Read the model definition and answer for the solid it produces. Units are mm, in the model's axes. Face numbers are marked on the shaded views. A direction names the side the tool comes from. Round coordinates to 2 decimals unless told otherwise and drop trailing zeros. Write each loop counter-clockwise with the first axis right and the second up, starting at its lowest first coordinate (ties: lowest second). Pieces come first, ordered by that corner, then holes. Notation, with made-up numbers: (81.25, -21) -> (127.25, -21) arc R19 ccw to (127.25, 1) -> close; hole circle Ø5 at (-0.5, -4.75). An arc over 180 degrees is marked (long way). Return JSON: item names as keys, results as strings.
from build123d import *

# Parameters (mm, degrees)
SKETCH1_R           = 2.75
SKETCH1_W           = 25
SKETCH1_H           = 18
BOSS_EXTRUDE1_DEPTH = 3
CUT_EXTRUDE1_REACH  = 132.035
SKETCH3_R           = 2.75
SKETCH2_R           = 2.75
BOSS_EXTRUDE2_DEPTH = 6
FILLET1_R           = 3
BOSS_EXTRUDE5_DEPTH = 4.5
BOSS_EXTRUDE6_DEPTH = 4.5


with BuildPart() as part:
    # Sketch1 → Boss-Extrude1 (new body)
    with BuildSketch(Plane.XY):
        Polygon((7.071067812, 0), (42.928932188, 0), (50, 7.071067812), (50, 43.5), (45.5, 48), (45.5, 112.928932188), (38.428932188, 120), (11.571067812, 120), (4.5, 112.928932188), (4.5, 48), (0, 43.5), (0, 7.071067812), align=None)
        with Locations((7.1, 10)):
            Circle(SKETCH1_R, mode=Mode.SUBTRACT)
        with Locations(Location((42.9, 10, 0), (0, 0, 180))):
            Circle(SKETCH1_R, mode=Mode.SUBTRACT)
        with BuildLine():
            Line((19, 50.75), (19, 104))
            ThreePointArc((19, 104), (25, 110), (31, 104))
            Line((31, 104), (31, 50.75))
            ThreePointArc((31, 50.75), (25, 44.75), (19, 50.75))
        make_face(mode=Mode.SUBTRACT)
        with Locations((25, 17.5)):
            Rectangle(SKETCH1_W, SKETCH1_H, mode=Mode.SUBTRACT)
    extrude(amount=BOSS_EXTRUDE1_DEPTH)

    # Sketch3 → Cut-Extrude1 (cut, up to next)
    with BuildSketch(Plane.XY.offset(3), mode=Mode.PRIVATE) as cut_extrude1_sk1:
        with Locations((15, 33)):
            Circle(SKETCH3_R)
    cut_extrude1_tool1 = extrude(cut_extrude1_sk1.sketch, amount=-CUT_EXTRUDE1_REACH, mode=Mode.PRIVATE) & part.part
    # Sketch3 → Cut-Extrude1 (cut, up to next)
    with BuildSketch(Plane.XY.offset(3), mode=Mode.PRIVATE) as cut_extrude1_sk2:
        with Locations((35, 33)):
            Circle(SKETCH3_R)
    cut_extrude1_tool2 = extrude(cut_extrude1_sk2.sketch, amount=-CUT_EXTRUDE1_REACH, mode=Mode.PRIVATE) & part.part
    add(cut_extrude1_tool1.solids().sort_by_distance((15, 33, 3))[0], mode=Mode.SUBTRACT)
    add(cut_extrude1_tool2.solids().sort_by_distance((35, 33, 3))[0], mode=Mode.SUBTRACT)

    # Sketch2 → Boss-Extrude2 (add)
    with BuildSketch(Plane(origin=(0, 0, 0), x_dir=(-1, 0, 0), z_dir=(0, 0, -1))):
        Polygon((-50, 18.19), (-37.5, 18.19), (-37.5, 26.5), (-12.5, 26.5), (-12.5, 18.19), (0, 18.19), (0, 43.5), (-4.5, 48), (-4.5, 112.928932188), (-9.5, 117.928932188), (-9.5, 40.75), (-40.5, 40.75), (-40.5, 117.928932188), (-45.5, 112.928932188), (-45.5, 48), (-50, 43.5), align=None)
        with Locations(Location((-35, 33, 0), (0, 0, 180))):
            Circle(SKETCH2_R, mode=Mode.SUBTRACT)
        with Locations(Location((-15, 33, 0), (0, 0, 180))):
            Circle(SKETCH2_R, mode=Mode.SUBTRACT)
    extrude(amount=BOSS_EXTRUDE2_DEPTH)

    # Fillet1
    fillet1_edges = [part.edges().sort_by_distance(p)[0] for p in [
        (37.5, 8.5, 1.5),
        (37.5, 26.5, -3),
        (12.5, 26.5, -3),
        (12.5, 8.5, 1.5),
    ]]
    fillet(fillet1_edges, radius=FILLET1_R)

    # Sketch4 → Boss-Extrude5 (add)
    with BuildSketch(Plane(origin=(45.5, 0, 0), x_dir=(0, 0, -1), z_dir=(1, 0, 0))):
        Polygon((-3, 43.5), (60.8, 43.5), (6, 112.928932188), (-3, 112.928932188), align=None)
    extrude(amount=BOSS_EXTRUDE5_DEPTH)

    # Sketch7 → Boss-Extrude6 (add)
    with BuildSketch(Plane.ZY.offset(-4.5)):
        Polygon((3, 112.928932188), (3, 43.5), (-60.8, 43.5), (-6, 112.928932188), align=None)
    extrude(amount=BOSS_EXTRUDE6_DEPTH)


solid = part.part
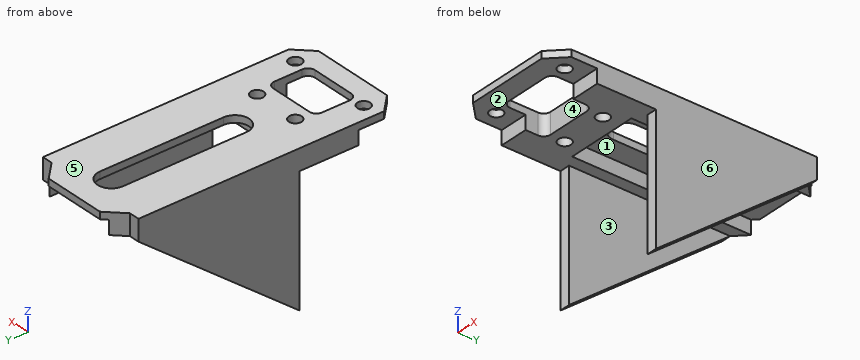
Item 1: Flat-ended cylindrical pins translate along their axes: pin 1 (2 mm diameter, centred on x = 38.5, z = -5.5, fed in from -Y); pin 2 (9.5 mm diameter, centred on x = 27.5, y = 84.5, fed in from -Z); pin 3 (3.5 mm diameter, centred on x = 2.5, z = -1.5, fed in from +Y). Find the tip coordinate at first contact, or state that the pin passes through.
Worked answers:
{"pin 1": "stops at y = 18.19", "pin 2": "stops at z = 0", "pin 3": "stops at y = 112.93"}
Item 2: Straight lines are drawn through the part: L1, parallel to X at y = 33, z = -1.5; L2, parallel to X at y = 51, z = -40; L3, parallel to Z at x = 11.5, y = 79.5. For each, find the intervals that lie inside material, in ascending order. Write a range as [from, to].
Worked answers:
{"L1": "x = [0, 12.25], [17.75, 32.25], [37.75, 50]", "L2": "x = [0, 4.5], [45.5, 50]", "L3": "z = [0, 3]"}
Item 3: Section D-D (y = 69) is taken. Give the vertices of the cut face in (x, z), then the cut area to 3 significant figures.
Worked answers:
{"outline": "(0, -40.67) -> (4.5, -40.67) -> (4.5, -6) -> (9.5, -6) -> (9.5, 0) -> (19, 0) -> (19, 3) -> (0, 3) -> close; (31, 0) -> (40.5, 0) -> (40.5, -6) -> (45.5, -6) -> (45.5, -40.67) -> (50, -40.67) -> (50, 3) -> (31, 3) -> close", "area": "540 mm2"}
Item 4: Section C-C (y = 97) is taken. Give the vertices of the cut face in (x, z), then the cut area to 3 significant figures.
Worked answers:
{"outline": "(0, -18.57) -> (4.5, -18.57) -> (4.5, -6) -> (9.5, -6) -> (9.5, 0) -> (19, 0) -> (19, 3) -> (0, 3) -> close; (31, 0) -> (40.5, 0) -> (40.5, -6) -> (45.5, -6) -> (45.5, -18.57) -> (50, -18.57) -> (50, 3) -> (31, 3) -> close", "area": "341 mm2"}
Item 5: Section A-A (y = 33) is taken. Give the vertices of the cut face in (x, z).
Worked answers:
{"outline": "(0, -6) -> (12.25, -6) -> (12.25, 3) -> (0, 3) -> close; (17.75, -6) -> (32.25, -6) -> (32.25, 3) -> (17.75, 3) -> close; (37.75, -6) -> (50, -6) -> (50, 3) -> (37.75, 3) -> close"}
Item 6: Section B-B (z = -23) is taken. Give the vertices of the cut face in (x, y), then the cut area to 3 significant figures.
Worked answers:
{"outline": "(0, 43.5) -> (4.5, 43.5) -> (4.5, 91.39) -> (0, 91.39) -> close; (45.5, 43.5) -> (50, 43.5) -> (50, 91.39) -> (45.5, 91.39) -> close", "area": "431 mm2"}
Item 7: For a pull along X with two mould halves and no side action, classify the marked faces 4, 5 and 6 as released by +X, released by -X, zero draft, split by the parting line, or undercut.
Worked answers:
{"face 4": "undercut", "face 5": "zero draft", "face 6": "released by +X"}
Item 8: A tool of negligible diameter and unlimited length cuts with its end or side. For the marked faces 1, 2 and 3, from which of +Z, -Z, +X, -X, +Y, -Y can it reach the whole face along a straight path? Write none if from no direction.
Worked answers:
{"face 1": "-Z, +Y", "face 2": "-Z, +X, -X, -Y", "face 3": "-Z, +Y, -Y"}
